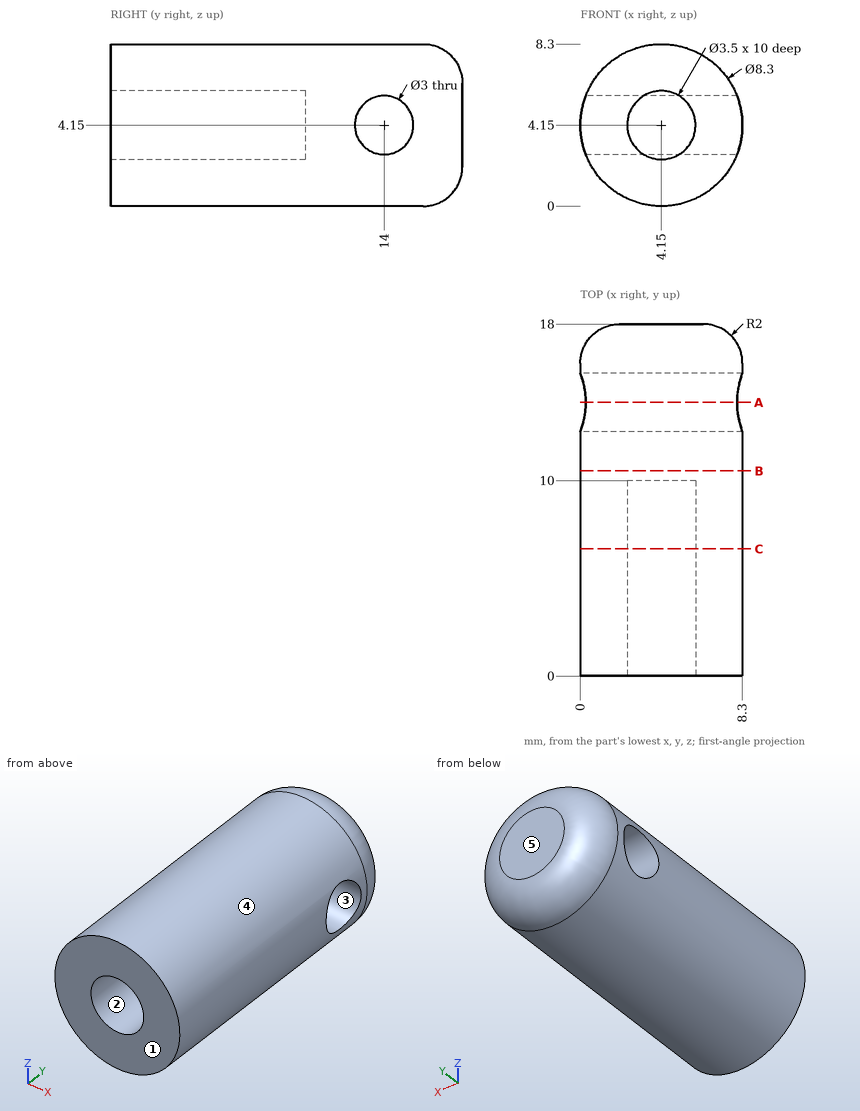
Part print with two shaded views. Sizes in mm from the minimum x, y, z corner. A direction names the side the tool comes from. Coordinates: 2 decimals unless noted, no trailing zeros. Write each loop counter-clockwise with the first axis right and the second up, starting at its lowest first coordinate (ties: lowest second). Pieces come first, ordered by that corner, then holes. Notation, with made-up numbers: (11, 73.25) - (33, 73.25) arc R32 ccw to (33, 101.25) - close; hole circle Ø2 at (31, 65). An arc over 180 degrees is marked (long way). Put each result on its own line as item: value.
1. Band-saw the part on C-C (y = 6.5). Write the cut outline in (x, z).
Final values:
outline: circle Ø8.3 at (4.15, 4.15); hole circle Ø3.5 at (4.15, 4.15)
2. 3-axis set-ups, long thin cutter, end or side, ignore diameter. For the marked faces 1 and 2: which of +Z, -Z, +X, -X, +Y, -Y reach the whole face in a straight line?
Final values:
face 1: +Z, -Z, +X, -X, -Y
face 2: -Y
3. Probe line 1 along X through (y, z) = (3.5, 4.15); line 2 along Y through (x, z) = (3.5, 4.15); line 3 along Y through (x, z) = (5.75, 5). List the from-to ranges inside material, lowest first. Write a range as [from, to].
Final values:
line 1: x = [0, 2.4], [5.9, 8.3]
line 2: y = [10, 12.5], [15.5, 18]
line 3: y = [0, 12.76], [15.24, 18]
4. Band-saw the part on B-B (y = 10.5). Write the cut outline in (x, z).
Final values:
outline: circle Ø8.3 at (4.15, 4.15)
5. Flat gauge pins, fed straight in: pin 1 Ø1 at (y, z) = (3.5, 2.5) entering from -X; pin 2 Ø1.8 at (x, z) = (4, 4.5) entering from -Y; pin 3 Ø2.5 at (y, z) = (14, 4.15) entering from +X; pin 4 Ø3 at (x, y) = (1, 12.5) entering from +Z. Where does each tip first touch, or does it go through?
Final values:
pin 1: stops at x = 0.16
pin 2: stops at y = 10
pin 3: passes through
pin 4: stops at z = 7.96
6. Band-saw the part on A-A (y = 14). Write the cut outline in (x, z).
Final values:
outline: (0.28, 2.65) arc R4.15 ccw to (8.02, 2.65) - close; (0.28, 5.65) - (8.02, 5.65) arc R4.15 ccw to start
7. Two-plate mould, pull along Z, no slides. Class the marked faces 3, 4 and 5: +Z half, -Z half, draft (parallel to the pull), parting line (faces both ways), or undercut.
Final values:
face 3: undercut
face 4: parting line
face 5: draft
